Print and shaded views of the part. All mm, measured from the part's lowest x, y and z. A direction names the side the tool comes from. Round coordinates to 2 decimals unless told otherwise and drop trailing zeros. Order: outer loops, then holes, each group sorted by start corner. A loop starts at its lowest first (then second) coordinate and runs counter-clockwise, first axis right, second up. Notation, with made-up numbers: (70, 42.5) - (84, 42.5) arc R33 cw to (84, 72.5) - close; hole circle Ø8 at (-6.75, -16). An arc over 180 degrees is marked (long way). Return JSON: item names as keys, results as strings. Group by question number.
Item 1: Saw through at D-D on z = 10.5. List the corners of the cut face in (x, y), and give its area (3 significant figures).
Item 2: Tool access for the marked faces 1 and 2: list every direction of +Z, -Z, +X, -X, +Y, -Y with a clear straight run to the whole face (end or side of a thin tool).
Item 3: Two-plate mould, pull along X, no slides. Class the marked faces 3, 4, 5 and 6: released by +X, released by -X, zero draft, split by the parting line, or undercut.
Item 4: Saw through at C-C on x = 1.5. List the corners of the cut face in (y, z).
Item 5: Saw through at A-A on y = 42.5. List the corners of the cut face in (x, z).
Item 6: Saw through at B-B on z = 6.35. State how many separate pieces and enclosed holes the cut face has.
Item 7: Probe probe 1 along Y at (x, z) = (21.7, 6.35) (1 decimal); probe 2 along X at (y, z) = (8, 12.25); probe 3 along Y at (x, z) = (3, 13.5). List the from-to ranges inside material, lowest first.
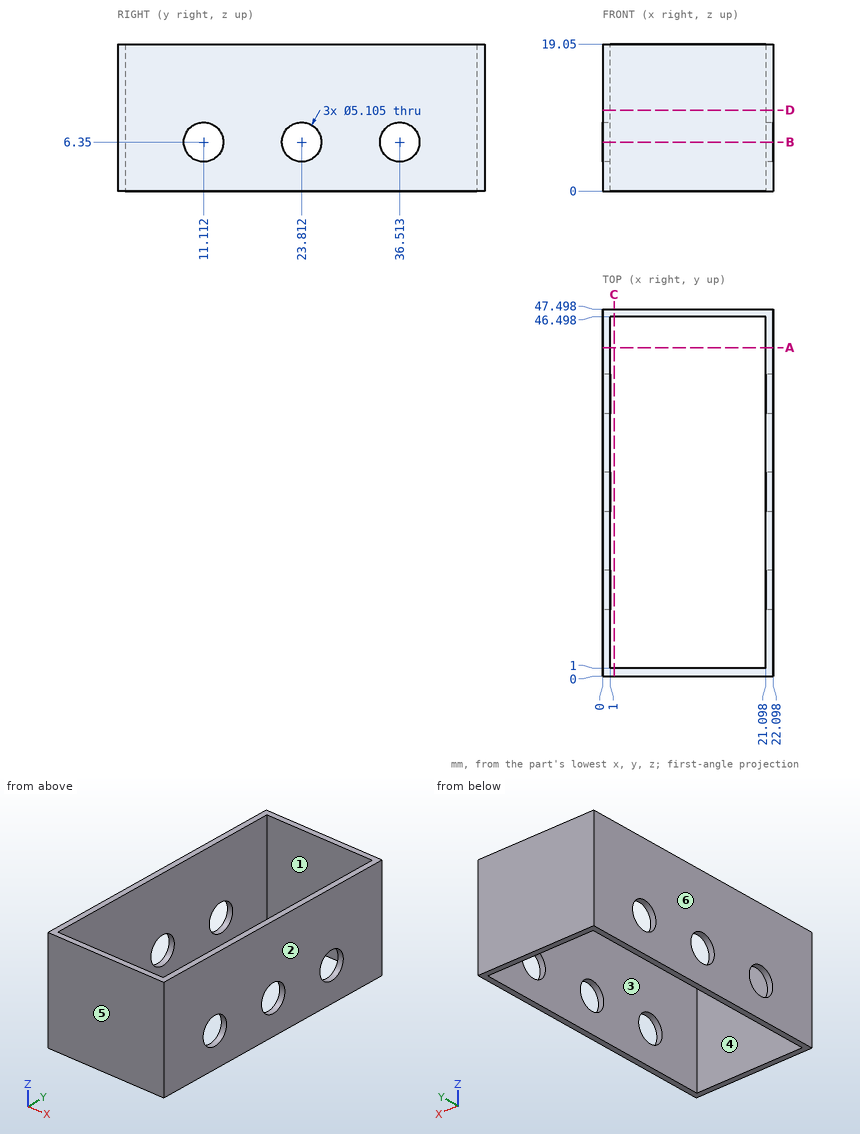
Filled in:
{
 "1": {"outline": "(0, 0) - (22.1, 0) - (22.1, 47.5) - (0, 47.5) - close; hole (1, 1) - (21.1, 1) - (21.1, 46.5) - (1, 46.5) - close", "area": "135 mm^2"},
 "2": {"face 1": "+Z, -Z", "face 2": "+Z, -Z, +X, +Y, -Y"},
 "3": {"face 3": "undercut", "face 4": "undercut", "face 5": "zero draft", "face 6": "released by -X"},
 "4": {"outline": "(0, 0) - (1, 0) - (1, 19.05) - (0, 19.05) - close; (46.5, 0) - (47.5, 0) - (47.5, 19.05) - (46.5, 19.05) - close"},
 "5": {"outline": "(0, 0) - (1, 0) - (1, 19.05) - (0, 19.05) - close; (21.1, 0) - (22.1, 0) - (22.1, 19.05) - (21.1, 19.05) - close"},
 "6": {"separate pieces": "6", "enclosed holes": "0"},
 "7": {"probe 1": "y = 0 to 8.6, 13.7 to 21.3, 26.4 to 34, 39.1 to 47.5", "probe 2": "x = 0 to 1, 21.1 to 22.1", "probe 3": "y = 0 to 1, 46.5 to 47.5"}
}
